Autodesk Inventor part; units mm, degrees
ref_plane "YZ Plane" through (0, 0, 0) normal (1, 0, 0) x (0, 1, 0)
ref_plane "XZ Plane" through (0, 0, 0) normal (0, 1, 0) x (-1, 0, 0)
ref_plane "XY Plane" through (0, 0, 0) normal (0, 0, 1) x (1, 0, 0)
sketch "스케치1" plane through (0, 0, 0) normal (0, 0, 1) x (1, 0, 0)
  line L0 (16.5, -19) -> (-16.5, -19)
  line L1 (-16.5, -19) -> (-16.5, 19)
  line L2 (-16.5, 19) -> (16.5, 19)
  line L3 (16.5, 19) -> (16.5, -19)
  line L4 (16.5, -19) -> (-16.5, 19) construction
  line L5 (-16.5, -19) -> (16.5, 19) construction
  line L6 (12.5, -14.5) -> (-12.5, -14.5)
  line L7 (-12.5, -14.5) -> (-12.5, 14.5)
  line L8 (-12.5, 14.5) -> (12.5, 14.5)
  line L9 (12.5, 14.5) -> (12.5, -14.5)
  line L10 (12.5, -14.5) -> (-12.5, 14.5) construction
  line L11 (-12.5, -14.5) -> (12.5, 14.5) construction
  circle A0 centre (-12.5, 14.5) radius 2
  circle A1 centre (12.5, 14.5) radius 2
  circle A2 centre (12.5, -14.5) radius 2
  circle A3 centre (-12.5, -14.5) radius 2
  point P0 (0, 0)
  dimension "d14" = 33
  dimension "d15" = 38
  dimension "d16" = 25
  dimension "d17" = 29
  dimension "d18" = 4
  dimension "d19" = 4
  dimension "d20" = 4
  dimension "d21" = 4
extrude "돌출1" add sketch "스케치1" along normal blind 1 contours L0 L1 L2 L3 | A3 L7 A0 L8 A1 L9 A2 L6
fillet "모깎기1" radius 2 4 edges at (-16.5, 19, 0.5) (16.5, 19, 0.5) (16.5, -19, 0.5) (-16.5, -19, 0.5)
sketch "스케치2" plane through (0, 0, 1) normal (0, 0, 1) x (1, 0, 0)
  circle A0 centre (0, 0) radius 5
  dimension "d11" = 10
extrude "돌출2" cut sketch "스케치2" against normal through all
properties part number "castor_top" material "알루미늄 6061"
Could you check a few things on this model? Use its own coordinates, in mm. Coordinates: 2 decimals unless noted, no trailing zeros. Order: outer loops, then holes, each group sorted by start corner. A loop starts at its lowest first (then second) coordinate and runs counter-clockwise, first axis right, second up. Notation, with made-up numbers: (8, 35.25) - (34, 35.25) arc R23 cw to (34, 47.25) - close; hole circle Ø5 at (32.5, 16.5). An arc over 180 degrees is marked (long way). Answer in a Markdown table with one row per item. Add a question column.
(1) If we section it at D-D, the plane x = 12.5: Please give me the cut outline in (y, z), then the cut area to 3 significant figures.
(2) I need wall thicknesses on L1, parallel to Y at x = -12.5, z = 0.2; L2, parallel to X at y = 14.5, z = 0.2; L3, parallel to Y at x = 13, z = 0.15. Which ranges of each line are inside material? Lowest first, please.
(3) Will this pin go through, and if not, where does the flat tip stop? pin 1 (6 mm diameter, centred on x = 0, y = 0, fed in from +Z).
(4) If we section it at A-A, the plane y = 0: Please give me the cut outline in (x, z), then the cut area to 3 significant figures.
(5) If we section it at C-C, the plane y = 14.5: Please give me the cut outline in (x, z), then the cut area to 3 significant figures.
(6) If we mould it in two halves opening along Y, with no side actions, what happens to faces 1 (the face through (-15.9, 18.43, 0.51)), 2 (the face through (-16.5, -0.2, 0.5)), 3 (the face through (-12.76, 12.517, 0.493))? For each: released by +Y, released by -Y, zero draft, split by the parting line, or undercut.
(7) If we section it at B-B, the plane x = 0: Please give me the cut outline in (y, z), then the cut area to 3 significant figures.
Results are:
| question | item | result |
|---|---|---|
| 1 | outline | (-19, 0) - (-16.5, 0) - (-16.5, 1) - (-19, 1) - close; (-12.5, 0) - (12.5, 0) - (12.5, 1) - (-12.5, 1) - close; (16.5, 0) - (19, 0) - (19, 1) - (16.5, 1) - close |
| 1 | area | 30.0 mm2 |
| 2 | L1 | y = -19 to -16.5, -12.5 to 12.5, 16.5 to 19 |
| 2 | L2 | x = -16.5 to -14.5, -10.5 to 10.5, 14.5 to 16.5 |
| 2 | L3 | y = -19 to -16.44, -12.56 to 12.56, 16.44 to 19 |
| 3 | pin 1 | passes through |
| 4 | outline | (-16.5, 0) - (-5, 0) - (-5, 1) - (-16.5, 1) - close; (5, 0) - (16.5, 0) - (16.5, 1) - (5, 1) - close |
| 4 | area | 23.0 mm2 |
| 5 | outline | (-16.5, 0) - (-14.5, 0) - (-14.5, 1) - (-16.5, 1) - close; (-10.5, 0) - (10.5, 0) - (10.5, 1) - (-10.5, 1) - close; (14.5, 0) - (16.5, 0) - (16.5, 1) - (14.5, 1) - close |
| 5 | area | 25.0 mm2 |
| 6 | face 1 | released by +Y |
| 6 | face 2 | zero draft |
| 6 | face 3 | undercut |
| 7 | outline | (-19, 0) - (-5, 0) - (-5, 1) - (-19, 1) - close; (5, 0) - (19, 0) - (19, 1) - (5, 1) - close |
| 7 | area | 28.0 mm2 |
